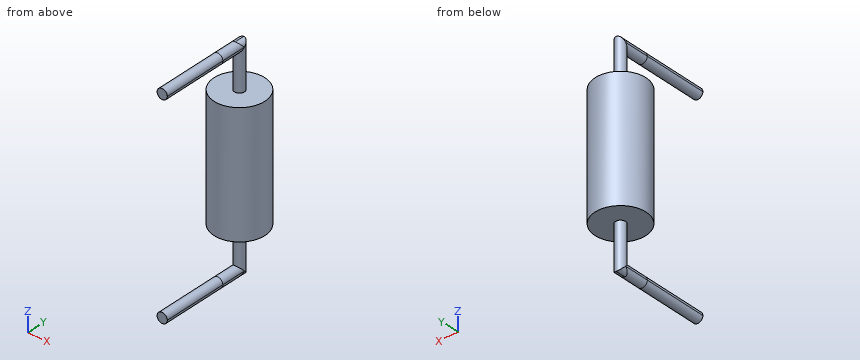
```python
from build123d import *

# Parameters (mm, degrees)
SKETCH1_R                       = 1.25
BOSS_EXTRUDE1_DEPTH             = 3
SKETCH2_R                       = 0.25
BOSS_EXTRUDE2_DEPTH             = 2.25
BOSS_EXTRUDE2_DEPTH_BACK        = 8.25
BOSS_EXTRUDE3_REACH             = 4.5
SKETCH3_R                       = 0.25
BOSS_EXTRUDE3_DIRECTION_2_DEPTH = 3.2
CUT_EXTRUDE1_DEPTH              = 6.7


with BuildPart() as part:
    # Sketch1 → Boss-Extrude1 (new body, symmetric)
    with BuildSketch(Plane.XY):
        with Locations((0, 1.25)):
            Circle(SKETCH1_R)
    extrude(amount=BOSS_EXTRUDE1_DEPTH, both=True)

    # Sketch2 → Boss-Extrude2 (add, two sides)
    with BuildSketch(Plane.XY.offset(3)) as boss_extrude2_sk:
        with Locations((0, 1.25)):
            Circle(SKETCH2_R)
    extrude(amount=BOSS_EXTRUDE2_DEPTH)
    extrude(boss_extrude2_sk.sketch, amount=-BOSS_EXTRUDE2_DEPTH_BACK)

    # Sketch3 → Boss-Extrude3 (add, up to next)
    with BuildSketch(Plane(origin=(0, 0, 0), x_dir=(1, 0, 0), z_dir=(0, 1, 0)), mode=Mode.PRIVATE) as boss_extrude3_sk1:
        with Locations((0, -5)):
            Circle(SKETCH3_R)
    boss_extrude3_tool1 = extrude(boss_extrude3_sk1.sketch, amount=BOSS_EXTRUDE3_REACH, mode=Mode.PRIVATE) - part.part
    add(boss_extrude3_tool1.solids().sort_by_distance((0, 0, 5))[0])
    # Sketch3 → Boss-Extrude3 (add, up to next)
    with BuildSketch(Plane(origin=(0, 0, 0), x_dir=(1, 0, 0), z_dir=(0, 1, 0)), mode=Mode.PRIVATE) as boss_extrude3_sk2:
        with Locations((0, 5)):
            Circle(SKETCH3_R)
    boss_extrude3_tool2 = extrude(boss_extrude3_sk2.sketch, amount=BOSS_EXTRUDE3_REACH, mode=Mode.PRIVATE) - part.part
    add(boss_extrude3_tool2.solids().sort_by_distance((0, 0, -5))[0])

    # Sketch3 → Boss-Extrude3 direction 2 (add)
    with BuildSketch(Plane(origin=(0, 0, 0), x_dir=(1, 0, 0), z_dir=(0, 1, 0))):
        with Locations((0, -5)):
            Circle(SKETCH3_R)
        with Locations((0, 5)):
            Circle(SKETCH3_R)
    extrude(amount=-BOSS_EXTRUDE3_DIRECTION_2_DEPTH)

    # Sketch4 → Cut-Extrude1 (cut, through all)
    with BuildSketch(Plane(origin=(0, -3.2, 0), x_dir=(-1, 0, 0), z_dir=(0, -1, 0))):
        with BuildLine():
            Line((0.25, -5), (0.35, -5))
            Line((0.35, -5), (0.35, -5.35))
            Line((0.35, -5.35), (-0.35, -5.35))
            Line((-0.35, -5.35), (-0.35, -5))
            Line((-0.35, -5), (-0.25, -5))
            ThreePointArc((-0.25, -5), (0, -5.25), (0.25, -5))
        make_face()
        with BuildLine():
            Line((-0.25, 5), (-0.35, 5))
            Line((-0.35, 5), (-0.35, 5.35))
            Line((-0.35, 5.35), (0.35, 5.35))
            Line((0.35, 5.35), (0.35, 5))
            Line((0.35, 5), (0.25, 5))
            ThreePointArc((0.25, 5), (0, 5.25), (-0.25, 5))
        make_face()
    extrude(amount=-CUT_EXTRUDE1_DEPTH, mode=Mode.SUBTRACT)


solid = part.part
```
Verification items for the finished model (mm, model axes). Give positions to 0.01 mm unless a question says otherwise; leave off trailing zeros. Loops run counter-clockwise (first coordinate to the right, second up) from the corner with the lowest first, then second, coordinate; pieces in that order, holes last.
1. Section check B-B, the plane z = -1. Enter the section's corners in (x, y), then the cut area to 3 significant figures.
2. Thickness scan on line 1 (Z direction, x = 0.3, y = 0.5); line 2 (X direction, y = 1.2, z = 1.25); line 3 (Z direction, x = 0.15, y = -0.9). Record the ranges inside material, lowest first.
3. Section check A-A, the plane y = 0.25. Enter the section's corners in (x, z), then the cut area to 3 significant figures.
4. Section check C-C, the plane x = 0.75. Enter the section's corners in (y, z), then the cut area to 3 significant figures.
5. Go/stop test with flat-tipped pins: pin 1 Ø1.5 at (y, z) = (-1, 0.5) entering from -X; pin 2 Ø1.5 at (x, y) = (-0.5, -2) entering from -Z; pin 3 Ø1 at (x, z) = (0, 1) entering from -Y. Record where each tip stops, or that it passes through.
6. Section check D-D, the plane y = -2.45. Enter the section's corners in (x, z).
Geometry says:
1. outline: circle Ø2.5 at (0, 1.25)
1. area: 4.91 mm2
2. line 1: z = -3 to 3
2. line 2: x = -1.25 to 1.25
2. line 3: z = -5.2 to -4.8, 4.8 to 5.2
3. outline: (-0.75, -3) - (0.75, -3) - (0.75, 3) - (-0.75, 3) - close; circle Ø0.5 at (0, -5); circle Ø0.5 at (0, 5)
3. area: 9.39 mm2
4. outline: (0.25, -3) - (2.25, -3) - (2.25, 3) - (0.25, 3) - close
4. area: 12.0 mm2
5. pin 1: passes through
5. pin 2: stops at z = -5.25
5. pin 3: stops at y = 0
6. outline: circle Ø0.5 at (0, -5); circle Ø0.5 at (0, 5)
